```python
from build123d import *

# Parameters (mm, degrees)
F1_DEPTH      = 25
F2_T1_DEPTH   = 79.8532648187
F4_DEPTH      = 25
F4_DEPTH_BACK = 25
F5_T1_DEPTH   = 107.1220330496
F7_DEPTH      = 25
F8_R          = 6.2148490945
F9_DEPTH      = 25
F9_DEPTH_BACK = 25
F10_R         = 7.2426406871


# Not quite as in the source:
# - a fillet or chamfer that OpenCascade refuses, or shapes differently, is made with other operations: its cross-section is extruded or revolved along the edge and cut away or added


with BuildPart() as f1:
    # F0 (on Front) → F1 (new body)
    with BuildSketch(Plane.XZ):
        Polygon((4.8560337164, 7.4956272729), (0, 7.4956272729), (-4.8560337164, 7.4956272729), (0, -16.87037386), align=None)
    extrude(amount=F1_DEPTH)

    # F2: fillet of radius 2.1864014695 on 1 edges, made by hand

    # F2_s2 → F2_t1 (cut)
    with BuildSketch(Plane.XZ.offset(-27.4266324093)):
        with BuildLine():
            ThreePointArc((-2.1442330518, -6.1113083304), (0, -7.87037386), (2.1442330518, -6.1113083304))
            Line((2.1442330518, -6.1113083304), (0, -16.87037386))
            Line((0, -16.87037386), (-2.1442330518, -6.1113083304))
        make_face()
    extrude(amount=F2_T1_DEPTH, mode=Mode.SUBTRACT)

    # F3 (on Right) → F4 (cut, two sides)
    with BuildSketch(Plane.YZ) as f4_sk:
        with BuildLine():
            ThreePointArc((1.5301647967, 9.1992565168), (-4.4063240448, -7.9303751627), (-16.6751330548, -21.2773788233))
            Line((-16.6751330548, -21.2773788233), (1.5301647967, -21.2773788233))
            Line((1.5301647967, -21.2773788233), (1.5301647967, 9.1992565168))
        make_face()
    extrude(amount=-F4_DEPTH, mode=Mode.SUBTRACT)
    extrude(f4_sk.sketch, amount=F4_DEPTH_BACK, mode=Mode.SUBTRACT)

    # F5: chamfer of 5.5 on 1 edges, made by hand

    # F5_s2 → F5_t1 (cut)
    with BuildSketch(Plane.YZ.offset(-53.5610165248)):
        with BuildLine():
            Line((0.079428002, 10.2204041802), (-9.7965992647, -15.2892315683))
            Line((-9.7965992647, -15.2892315683), (-9.7152756624, -15.3633022893))
            ThreePointArc((-9.7152756624, -15.3633022893), (-3.8594523105, -7.2118040219), (0.1053121044, 2.0189976591))
            Line((0.1053121044, 2.0189976591), (0.11, 2.0507680961))
            ThreePointArc((0.11, 2.0507680961), (0.11, 6.1355861381), (0.189428002, 10.2204041802))
            Line((0.189428002, 10.2204041802), (0.079428002, 10.2204041802))
        make_face()
    extrude(amount=F5_T1_DEPTH, mode=Mode.SUBTRACT)

    # F6 (on face) → F7 (cut)
    with BuildSketch(Plane.XY.offset(7.4956272729)):
        Polygon((7.9051312059, 6.1967439927), (-4.8560337164, -0.9754663641), (7.9051312059, -15.5989079942), align=None)
    extrude(amount=-F7_DEPTH, mode=Mode.SUBTRACT)

    # F8 (on Right) → F9 (cut, two sides)
    with BuildSketch(Plane.YZ) as f9_sk:
        with Locations((-17.4094103277, 0.4502551164)):
            Circle(F8_R)
    extrude(amount=F9_DEPTH, mode=Mode.SUBTRACT)
    extrude(f9_sk.sketch, amount=-F9_DEPTH_BACK, mode=Mode.SUBTRACT)

    # F10
    f10_edges = [f1.edges().sort_by_distance(p)[0] for p in [
        (0, -25, 7.495627),
    ]]
    fillet(f10_edges, radius=F10_R)


solid = f1.part
```
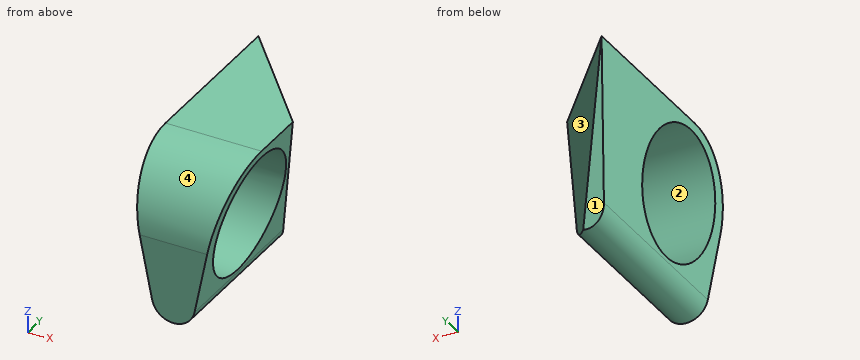
Model file for the job. Use its own axes, mm. Face numbers are marked on the shaded views. Coordinates: 2 decimals unless noted, no trailing zeros. Write each loop counter-clockwise with the first axis right and the second up, starting at its lowest first coordinate (ties: lowest second). Pieces come first, ordered by that corner, then holes. Notation, with made-up numbers: (7.25, -12.5) - (63.25, -12.5) arc R33 cw to (63.25, 25.5) - close; hole circle Ø5 at (-27.75, -30.5). An arc over 180 degrees is marked (long way). Use a Markdown table: item, result. Add a question column.
Item 1: Band-saw the part on B-B, the plane y = -15. Write the cut outline in (x, z).
Item 2: Drill centre lines: line 1 along Y through (x, z) = (1.5, -0.5); line 2 along Y through (x, z) = (1.5, -3.75); line 3 along Z through (x, y) = (4, -15). Where is each one in solid material? Low to high.
Item 3: Band-saw the part on A-A, the plane z = -3.5. Write the cut outline in (x, y).
Item 4: Drop flat-ended pins along their axis: pin 1 (3 mm diameter, centred on y = -11.5, z = -2.5, fed in from +X); pin 2 (3 mm diameter, centred on y = -4, z = -3.5, fed in from -X); pin 3 (3 mm diameter, centred on x = 0, z = 3, fed in from +Y). Give the stop position or say it passes through.
Item 5: Two-plate mould, pull along Z, no slides. Class the marked faces 1, 2, 3 and 4: pulls with the +Z half, pulls with the -Z half, needs draft (parallel to the pull), parting line crosses it, or undercut.
Item 6: Band-saw the part on D-D, the plane z = 2.75. Write the cut outline in (x, y), and give its area (3 significant figures).
Item 7: Band-saw the part on C-C, the plane x = -1. Write the cut outline in (y, z).
A:
| question | item | result |
|---|---|---|
| 1 | outline | (-4.86, 7.5) - (-4.59, 6.18) - (4.59, 6.18) - (4.86, 7.5) - close; (-2.31, -5.28) - (-2.14, -6.11) arc R2.19 ccw to (2.14, -6.11) - (2.31, -5.28) - close |
| 2 | line 1 | y = -25 to -23.55, -11.27 to -8.26 |
| 2 | line 2 | y = -25 to -21.99, -12.83 to -8.26 |
| 2 | line 3 | z = 6.18 to 7.5 |
| 3 | outline | (-2.66, -25) - (2.66, -25) - (2.66, -22.21) - (-2.66, -22.21) - close; (-2.66, -12.61) - (2.66, -12.61) - (2.66, -9.59) - (-1.14, -5.23) - (-2.66, -5.23) - close |
| 4 | pin 1 | stops at x = 3.16 |
| 4 | pin 2 | stops at x = -2.93 |
| 4 | pin 3 | stops at y = -4.82 |
| 5 | face 1 | pulls with the -Z half |
| 5 | face 2 | undercut |
| 5 | face 3 | needs draft |
| 5 | face 4 | pulls with the +Z half |
| 6 | outline | (-3.91, -24.56) - (3.91, -24.56) - (3.91, -23.18) - (-3.91, -23.18) - close; (-3.91, -11.64) - (3.91, -11.64) - (3.91, -11.02) - (-3.25, -2.81) - (-3.91, -2.81) - close |
| 6 | area | 50.3 mm² |
| 7 | outline | (-25, -7.63) - (-6.83, -7.63) - (-5.39, -3.92) - (-5.39, 7.5) - (-17.76, 7.5) arc R7.24 ccw to (-25, 0.25) - close; hole circle Ø12.43 at (-17.41, 0.45) |
